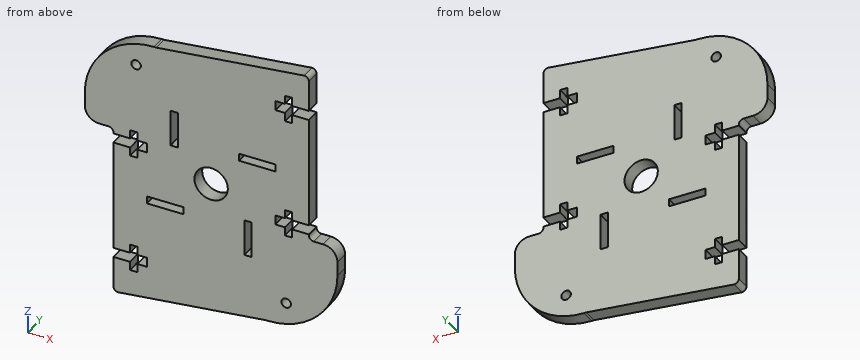
```python
from build123d import *

# Parameters (mm, degrees)
ESBO_O1_W                = 53
ESBO_O1_H                = 60
RESSALTO_EXTRUS_O1_DEPTH = 3
ESBO_O4_W                = 1.55
ESBO_O4_H                = 7.65
ESBO_O4_W_2              = 7.65
ESBO_O4_H_2              = 1.55
CORTE_EXTRUS_O2_DEPTH    = 10
ESBO_O5_R                = 1
CORTE_EXTRUS_O3_DEPTH    = 41.140378673
ESBO_O7_R                = 3.5
CORTE_EXTRUS_O6_DEPTH    = 41.140378673
ESBO_O8_W                = 6
ESBO_O8_H                = 36
CORTE_EXTRUS_O7_DEPTH    = 41.140378673
FILETE2_R                = 3
FILETE3_R                = 1
CORTE_EXTRUS_O8_DEPTH    = 41.140378673
CORTE_EXTRUS_O9_DEPTH    = 41.140378673


with BuildPart() as part:
    # Esboço1 → Ressalto-extrusão1 (new body)
    with BuildSketch(Plane(origin=(0, 0, 0), x_dir=(1, 0, 0), z_dir=(0, 1, 0))):
        Rectangle(ESBO_O1_W, ESBO_O1_H)
    extrude(amount=RESSALTO_EXTRUS_O1_DEPTH)

    # Esboço4 → Corte-extrusão2 (cut)
    with BuildSketch(Plane(origin=(0, 3, 0), x_dir=(-1, 0, 0), z_dir=(0, 1, 0))):
        with Locations((-7.725, -9.675)):
            Rectangle(ESBO_O4_W, ESBO_O4_H)
        with Locations((-9.675, 7.725)):
            Rectangle(ESBO_O4_W_2, ESBO_O4_H_2)
        with Locations((7.725, 9.675)):
            Rectangle(ESBO_O4_W, ESBO_O4_H)
        with Locations((9.675, -7.725)):
            Rectangle(ESBO_O4_W_2, ESBO_O4_H_2)
    extrude(amount=-CORTE_EXTRUS_O2_DEPTH, mode=Mode.SUBTRACT)

    # Esboço5 → Corte-extrusão3 (cut, through all)
    with BuildSketch(Plane(origin=(0, 3, 0), x_dir=(1, 0, 0), z_dir=(0, 1, 0))):
        with Locations(Location((-15.742640687, -21.399494937, 0), (0, 0, 270))):
            Circle(ESBO_O5_R)
        with Locations(Location((15.742640687, 21.399494937, 0), (0, 0, 270))):
            Circle(ESBO_O5_R)
    extrude(amount=-CORTE_EXTRUS_O3_DEPTH, mode=Mode.SUBTRACT)

    # Esboço7 → Corte-extrusão6 (cut, through all)
    with BuildSketch(Plane(origin=(0, 3, 0), x_dir=(1, 0, 0), z_dir=(0, 1, 0))):
        with Locations(Location((0, 0, 0), (0, 0, 270))):
            Circle(ESBO_O7_R)
    extrude(amount=-CORTE_EXTRUS_O6_DEPTH, mode=Mode.SUBTRACT)

    # Esboço8 → Corte-extrusão7 (cut, through all)
    with BuildSketch(Plane(origin=(0, 3, 0), x_dir=(1, 0, 0), z_dir=(0, 1, 0))):
        with Locations((23.5, -12)):
            Rectangle(ESBO_O8_W, ESBO_O8_H)
        with Locations((-23.5, 12)):
            Rectangle(ESBO_O8_W, ESBO_O8_H)
    extrude(amount=-CORTE_EXTRUS_O7_DEPTH, mode=Mode.SUBTRACT)

    # Filete2
    filete2_edges = [part.edges().sort_by_distance(p)[0] for p in [
        (26.5, 1.5, -6),
        (-26.5, 1.5, 6),
    ]]
    fillet(filete2_edges, radius=FILETE2_R)

    # Filete3
    filete3_edges = [part.edges().sort_by_distance(p)[0] for p in [
        (20.5, 1.5, 30),
        (20.5, 1.5, -6),
        (-20.5, 1.5, -30),
        (-20.5, 1.5, 6),
    ]]
    fillet(filete3_edges, radius=FILETE3_R)

    # Esboço9 → Corte-extrusão8 (cut, through all)
    with BuildSketch(Plane(origin=(0, 3, 0), x_dir=(1, 0, 0), z_dir=(0, 1, 0))):
        Polygon((-13.5, 20.5), (-15.5, 20.5), (-15.5, 18.7), (-17, 18.7), (-17, 20.5), (-20.5, 20.5), (-20.5, 22.5), (-17, 22.5), (-17, 24.3), (-15.5, 24.3), (-15.5, 22.5), (-13.5, 22.5), align=None)
        Polygon((-13.5, -4.74347437), (-15.5, -4.74347437), (-15.5, -6.54347437), (-17, -6.54347437), (-17, -4.74347437), (-20.5, -4.74347437), (-20.5, -2.74347437), (-17, -2.74347437), (-17, -0.94347437), (-15.5, -0.94347437), (-15.5, -2.74347437), (-13.5, -2.74347437), align=None)
        Polygon((13.5, -20.5), (15.5, -20.5), (15.5, -18.7), (17, -18.7), (17, -20.5), (20.5, -20.5), (20.5, -22.5), (17, -22.5), (17, -24.3), (15.5, -24.3), (15.5, -22.5), (13.5, -22.5), align=None)
        Polygon((13.5, 4.74347437), (15.5, 4.74347437), (15.5, 6.54347437), (17, 6.54347437), (17, 4.74347437), (20.5, 4.74347437), (20.5, 2.74347437), (17, 2.74347437), (17, 0.94347437), (15.5, 0.94347437), (15.5, 2.74347437), (13.5, 2.74347437), align=None)
    extrude(amount=-CORTE_EXTRUS_O8_DEPTH, mode=Mode.SUBTRACT)

    # Esboço10 → Corte-extrusão9 (cut, through all)
    with BuildSketch(Plane(origin=(0, 3, 0), x_dir=(1, 0, 0), z_dir=(0, 1, 0))):
        with BuildLine():
            Line((26.5, 11.5), (26.5, 12))
            ThreePointArc((26.5, 12), (22.253048327, 22.253048327), (12, 26.5))
            Line((12, 26.5), (11.5, 26.5))
            Line((11.5, 26.5), (-19.5, 30))
            Line((-19.5, 30), (-19.5, 39.997592749))
            Line((-19.5, 39.997592749), (32.53430666, 39.997592749))
            Line((32.53430666, 39.997592749), (32.53430666, 11.5))
            Line((32.53430666, 11.5), (26.5, 11.5))
        make_face()
        with BuildLine():
            Line((-26.5, -11.5), (-26.5, -12))
            ThreePointArc((-26.5, -12), (-22.253048327, -22.253048327), (-12, -26.5))
            Line((-12, -26.5), (-11.5, -26.5))
            Line((-11.5, -26.5), (19.5, -30))
            Line((19.5, -30), (19.5, -39.997592749))
            Line((19.5, -39.997592749), (-32.53430666, -39.997592749))
            Line((-32.53430666, -39.997592749), (-32.53430666, -11.5))
            Line((-32.53430666, -11.5), (-26.5, -11.5))
        make_face()
    extrude(amount=-CORTE_EXTRUS_O9_DEPTH, mode=Mode.SUBTRACT)


solid = part.part
```
Can you work these out from the model? Positions are in its coordinate system, mm. Round coordinates to 2 decimals unless told otherwise and drop trailing zeros. Loops run counter-clockwise (first coordinate to the right, second up) from the corner with the lowest first, then second, coordinate; pieces in that order, holes last. Notation, with made-up numbers: M 89.5,-13 L 141.5,-13 A32 cw 141.5,17 Z; hole C 2.5,64 d9. An arc over 180 degrees is marked long. Write item = value, one per line. Start each with the question number.
(1) I'm going to push flat-ended pins straight in: P1, Ø0.5, axis at y = 2, z = -23.5, coming from the -X side; P2, Ø0.5, axis at y = 1.5, z = 23.5, coming from the +X side; P3, Ø0.8, axis at x = 7.5, y = 1.5, coming from the +Z side. Where does each tip first touch, or does it pass through?
(2) Suppose I cut it at B-B on x = 0. Write out the boundary of the cut face in (y, z).
(3) Suppose I cut it at D-D on z = 16. Write out the boundary of the cut face in (x, y), plus the area to 3 significant figures.
(4) I need wall thicknesses on line 1 along X through (y, z) = (2.5, 5); line 2 along Z through (x, y) = (20, 1.95); line 3 along Z through (x, y) = (17.5, 0.45). Which ranges of each line are inside material? Lowest first, please.
(5) Suppose I cut it at A-A on z = 0. Write out the boundary of the cut face in (x, y).
(6) Suppose I cut it at C-C on y = 1.45. Give the number of separate pieces and of enclosed holes in the cut face, plus the area to 3 significant figures.
Answer block:
q1.P1 = -20.5
q1.P2 = 20.5
q1.P3 = 28.69
q2.outline = M 0,-27.8 L 3,-27.8 L 3,-3.5 L 0,-3.5 Z; M 0,3.5 L 3,3.5 L 3,27.8 L 0,27.8 Z
q3.outline = M -25.94,0 L 20.5,0 L 20.5,3 L -25.94,3 Z
q3.area = 139 mm²
q4.line_1 = -20.5 to -17, -15.5 to 20.5
q4.line_2 = -24.09 to -4.74, -2.74 to 20.5, 22.5 to 29.87
q4.line_3 = -25.42 to -4.74, -2.74 to 20.5, 22.5 to 29.77
q5.outline = M -20.5,0 L -3.5,0 L -3.5,3 L -20.5,3 Z; M 3.5,0 L 20.5,0 L 20.5,3 L 3.5,3 Z
q6.separate_pieces = 1
q6.enclosed_holes = 7
q6.area = 2,270 mm²
